```python
from build123d import *

# Parameters (mm, degrees)
SKETCH1_W           = 215.9
SKETCH1_H           = 234.95
BOSS_EXTRUDE1_DEPTH = 41.275
FILLET1_R           = 19.05
CUT_EXTRUDE1_REACH  = 323.742
SKETCH3_R           = 26.9875
CUT_EXTRUDE2_DEPTH  = 13.97
FILLET2_R           = 19.05


with BuildPart() as part:
    # Sketch1 → Boss-Extrude1 (new body)
    with BuildSketch(Plane(origin=(0, 0, 0), x_dir=(1, 0, 0), z_dir=(0, 1, 0))):
        with Locations((107.95, 117.475)):
            Rectangle(SKETCH1_W, SKETCH1_H)
    extrude(amount=BOSS_EXTRUDE1_DEPTH)

    # Fillet1
    fillet1_edges = [part.edges().sort_by_distance(p)[0] for p in [
        (0, 20.6375, -234.95),
        (215.9, 20.6375, -234.95),
        (215.9, 20.6375, 0),
        (0, 20.6375, 0),
    ]]
    fillet(fillet1_edges, radius=FILLET1_R)

    # Sketch3 → Cut-Extrude1 (cut, up to next)
    with BuildSketch(Plane(origin=(0, 41.275, 0), x_dir=(1, 0, 0), z_dir=(0, 1, 0)), mode=Mode.PRIVATE) as cut_extrude1_sk1:
        with Locations(Location((107.95, 195.2625, 0), (0, 0, 270))):
            Circle(SKETCH3_R)
    cut_extrude1_tool1 = extrude(cut_extrude1_sk1.sketch, amount=-CUT_EXTRUDE1_REACH, mode=Mode.PRIVATE) & part.part
    add(cut_extrude1_tool1.solids().sort_by_distance((107.95, 41.275, -195.2625))[0], mode=Mode.SUBTRACT)

    # Sketch4 → Cut-Extrude2 (cut)
    with BuildSketch(Plane(origin=(0, 41.275, 0), x_dir=(1, 0, 0), z_dir=(0, 1, 0))):
        with BuildLine():
            Line((215.9, 79.6925), (0, 79.6925))
            Line((0, 79.6925), (0, 215.9))
            ThreePointArc((0, 215.9), (5.579615818, 229.370384182), (19.05, 234.95))
            Line((19.05, 234.95), (196.85, 234.95))
            ThreePointArc((196.85, 234.95), (210.320384182, 229.370384182), (215.9, 215.9))
            Line((215.9, 215.9), (215.9, 79.6925))
        make_face()
    extrude(amount=-CUT_EXTRUDE2_DEPTH, mode=Mode.SUBTRACT)

    # Fillet2
    fillet2_edges = [part.edges().sort_by_distance(p)[0] for p in [
        (215.9, 34.29, -79.6925),
        (0, 34.29, -79.6925),
    ]]
    fillet(fillet2_edges, radius=FILLET2_R)


solid = part.part
```
Design review of the part built by this model. Coordinates are the model's own, in mm. A direction names the side the tool comes from. Coordinates: 2 decimals unless noted, no trailing zeros. Order: outer loops, then holes, each group sorted by start corner. A loop starts at its lowest first (then second) coordinate and runs counter-clockwise, first axis right, second up. Notation, with made-up numbers: (86.5, -26.75) -> (115.5, -26.75) arc R22 ccw to (115.5, -8.75) -> close; hole circle Ø11 at (16.25, 80.5). An arc over 180 degrees is marked (long way). One line per item, written item: value. Start each with the question number.
Q1. Mouldability with a two-part tool opening along X and no side actions: class faces 6 (the flat face through (106, 41.275, -40)), 7 (the cylindrical face through (91.53, 13.84, -216.68)), 8 (the cylindrical face through (5.43, 13.84, -229.22)), 9 (the flat face through (215.9, 16, -116)) as pulls with the +X half, pulls with the -X half, needs draft (parallel to the pull), parting line crosses it, or undercut.
Q2. Take a section at C-C, the plane y = 34.5. State the section outline as (x, z) points, then the cut area to 3 significant figures.
Q3. Insertion check: pin 1 Ø11 at (x, y) = (145.5, 31) entering from -Z; pin 2 Ø1 at (x, y) = (160, 35.5) entering from -Z; pin 3 Ø2 at (y, z) = (28.5, -182) entering from +X. Each pin has a flat end and moves straight along its axis. Give the tip position at first contact, or say it passes through.
Q4. Tool access review of faces 1 (the flat face through (109, 34, -79.692)), 2 (the cylindrical face through (210.17, 34.19, -74.26)), 3 (the flat face through (106, 0, -119)), 4 (the cylindrical face through (5.43, 34.19, -73.96)), 5 (the cylindrical face through (210.47, 13.84, -229.22)): name each direction out of +Z, -Z, +X, -X, +Y, -Y from which nothing blocks a thin tool from reaching the whole face with its end or side.
Q5. Take a section at D-D, the plane z = -77. State the section outline as (x, y) points (3 decimals), then the cut area to 3 significant figures.
Q6. For probe 1 along Z at (x, y) = (107, 19); probe 2 along Z at (x, y) = (74, 27.5); probe 3 along Y at (x, z) = (74, -107.5) (3 decimals), list the stretches that pass through material, from the lowest coordinate up.
Values follow:
1. face 6: needs draft
1. face 7: undercut
1. face 8: pulls with the -X half
1. face 9: pulls with the +X half
2. outline: (0, -60.64) arc R19.05 ccw to (19.05, -79.69) -> (196.85, -79.69) arc R19.05 ccw to (215.9, -60.64) -> (215.9, -19.05) arc R19.05 ccw to (196.85, 0) -> (19.05, 0) arc R19.05 ccw to (0, -19.05) -> close
2. area: 16,900 mm2
3. pin 1: stops at z = -234.95
3. pin 2: stops at z = -79.69
3. pin 3: passes through
4. face 1: -Z, +X, -X, +Y
4. face 2: -Z, +X, +Y
4. face 3: +Z, -Z, +X, -X, -Y
4. face 4: -Z, -X, +Y
4. face 5: -Z, +X, +Y, -Y
5. outline: (0, 0) -> (215.9, 0) -> (215.9, 27.305) -> (206.614, 27.305) -> (206.614, 41.275) -> (9.286, 41.275) -> (9.286, 27.305) -> (0, 27.305) -> close
5. area: 8,650 mm2
6. probe 1: z = -234.95 to -222.23, -168.29 to 0
6. probe 2: z = -79.69 to 0
6. probe 3: y = 0 to 27.305
